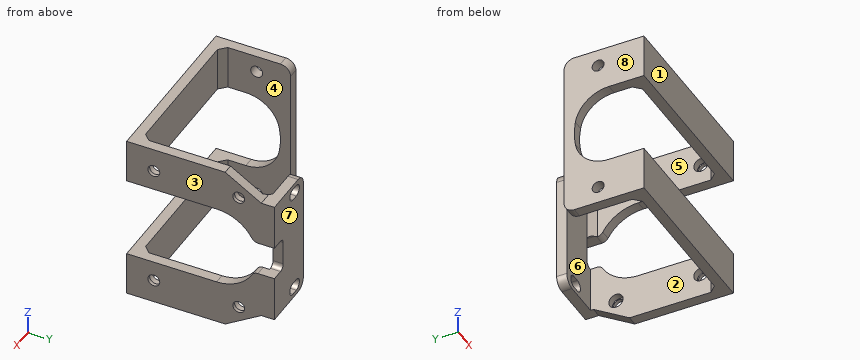
from build123d import *

# Parameters (mm, degrees)
EXTRUDE_THIN1_DEPTH = 25
SKETCH2_R           = 1.75
CUT_EXTRUDE1_DEPTH  = 3
CUT_EXTRUDE2_REACH  = 63.467
CUT_EXTRUDE3_REACH  = 63.467
CUT_EXTRUDE4_DEPTH  = 3
CUT_EXTRUDE5_REACH  = 72.48
SKETCH7_R           = 1.75
FILLET1_R           = 3
CUT_EXTRUDE7_REACH  = 63.467
SKETCH9_R           = 1.75
CUT_EXTRUDE8_START  = -3
CUT_EXTRUDE8_DEPTH  = 3
SKETCH11_R          = 2.1
CUT_EXTRUDE10_DEPTH = 2
CUT_EXTRUDE11_DEPTH = 10
CHAMFER1_SIZE       = 2
FILLET2_R           = 2


with BuildPart() as part:
    # Sketch1 → Extrude-Thin1 (new, symmetric)
    with BuildSketch(Plane.XY):
        Polygon((-1.5, 0), (-1.5, -23.5), (49.5, -23.5), (49.5, 20), (33, 20), (33, 17), (46.5, 17), (46.5, -20.5), (1.5, -20.5), (1.5, 0), align=None)
    extrude(amount=EXTRUDE_THIN1_DEPTH, both=True)

    # Sketch2 → Cut-Extrude1 (cut)
    with BuildSketch(Plane.ZY.offset(1.5)):
        with Locations(Location((-20, -10, 0), (0, 0, 270))):
            Circle(SKETCH2_R)
        with Locations(Location((20, -10, 0), (0, 0, 270))):
            Circle(SKETCH2_R)
    extrude(amount=-CUT_EXTRUDE1_DEPTH, mode=Mode.SUBTRACT)

    # Cut-Extrude2: up to this face of the body (flat: up to its plane)
    cut_extrude2_end = Plane(part.part.faces().sort_by_distance((46.5, -1.75, 0))[0])
    # Sketch3 → Cut-Extrude2 (cut, up to the picked face)
    with BuildSketch(Plane.ZY.offset(1.5), mode=Mode.PRIVATE) as cut_extrude2_sk1:
        with BuildLine():
            Line((-12, -13.167840434), (-12, -27.818696))
            Line((-12, -27.818696), (12, -27.818696))
            Line((12, -27.818696), (12, -13.167840434))
            ThreePointArc((12, -13.167840434), (9.637626158, -6.71286819), (3.666666667, -3.307707462))
            ThreePointArc((3.666666667, -3.307707462), (0, -3), (-3.666666667, -3.307707462))
            ThreePointArc((-3.666666667, -3.307707462), (-9.637626158, -6.71286819), (-12, -13.167840434))
        make_face()
    cut_extrude2_tool1 = split(extrude(cut_extrude2_sk1.sketch, amount=-CUT_EXTRUDE2_REACH, mode=Mode.PRIVATE), bisect_by=cut_extrude2_end, keep=Keep.BOTH, mode=Mode.PRIVATE)
    add(cut_extrude2_tool1.solids().sort_by(Axis((-1.5, -16.267413, 0), (1, 0, 0)))[0], mode=Mode.SUBTRACT)

    # Sketch5 → Cut-Extrude3 (cut, up to next)
    with BuildSketch(Plane(origin=(49.5, 0, 0), x_dir=(0, 0, -1), z_dir=(1, 0, 0)), mode=Mode.PRIVATE) as cut_extrude3_sk1:
        Polygon((-18.5, 20), (-18.5, 16.133851182), (-25, 5.502473915), (-25, 20), align=None)
    cut_extrude3_tool1 = extrude(cut_extrude3_sk1.sketch, amount=-CUT_EXTRUDE3_REACH, mode=Mode.PRIVATE) & part.part
    cut_extrude3 = cut_extrude3_tool1.solids().sort_by_distance((49.5, 14.896175, 22.37718))[0]
    add(cut_extrude3, mode=Mode.SUBTRACT)

    # Mirror1: Cut-Extrude3 across plane
    add(cut_extrude3.mirror(Plane.XY), mode=Mode.SUBTRACT)

    # Sketch6 → Cut-Extrude4 (cut)
    with BuildSketch(Plane(origin=(49.5, 0, 0), x_dir=(0, 0, -1), z_dir=(1, 0, 0))):
        with BuildLine():
            Line((-12, -23.5), (12, -23.5))
            Line((12, -23.5), (12, 3))
            ThreePointArc((12, 3), (0, 15), (-12, 3))
            Line((-12, 3), (-12, -23.5))
        make_face()
    extrude(amount=-CUT_EXTRUDE4_DEPTH, mode=Mode.SUBTRACT)

    # Sketch7 → Cut-Extrude5 (cut, up to next)
    with BuildSketch(Plane(origin=(0, 20, 0), x_dir=(1, 0, 0), z_dir=(0, 1, 0)), mode=Mode.PRIVATE) as cut_extrude5_sk1:
        with Locations(Location((38, 15.5, 0), (0, 0, 180))):
            Circle(SKETCH7_R)
    cut_extrude5_tool1 = extrude(cut_extrude5_sk1.sketch, amount=-CUT_EXTRUDE5_REACH, mode=Mode.PRIVATE) & part.part
    # Sketch7 → Cut-Extrude5 (cut, up to next)
    with BuildSketch(Plane(origin=(0, 20, 0), x_dir=(1, 0, 0), z_dir=(0, 1, 0)), mode=Mode.PRIVATE) as cut_extrude5_sk2:
        with Locations(Location((38, -15.5, 0), (0, 0, 180))):
            Circle(SKETCH7_R)
    cut_extrude5_tool2 = extrude(cut_extrude5_sk2.sketch, amount=-CUT_EXTRUDE5_REACH, mode=Mode.PRIVATE) & part.part
    add(cut_extrude5_tool1.solids().sort_by_distance((38, 20, -15.5))[0], mode=Mode.SUBTRACT)
    add(cut_extrude5_tool2.solids().sort_by_distance((38, 20, 15.5))[0], mode=Mode.SUBTRACT)

    # Fillet1
    fillet1_edges = [part.edges().sort_by_distance(p)[0] for p in [
        (0, 0, 25),
        (33, 18.5, 18.5),
        (0, 0, -25),
        (33, 18.5, -18.5),
    ]]
    fillet(fillet1_edges, radius=FILLET1_R)

    # Sketch9 → Cut-Extrude7 (cut, up to next)
    with BuildSketch(Plane(origin=(49.5, 0, 0), x_dir=(0, 0, -1), z_dir=(1, 0, 0)), mode=Mode.PRIVATE) as cut_extrude7_sk1:
        with Locations((-18, -15.5)):
            Circle(SKETCH9_R)
    cut_extrude7_tool1 = extrude(cut_extrude7_sk1.sketch, amount=-CUT_EXTRUDE7_REACH, mode=Mode.PRIVATE) & part.part
    # Sketch9 → Cut-Extrude7 (cut, up to next)
    with BuildSketch(Plane(origin=(49.5, 0, 0), x_dir=(0, 0, -1), z_dir=(1, 0, 0)), mode=Mode.PRIVATE) as cut_extrude7_sk2:
        with Locations((18, -15.5)):
            Circle(SKETCH9_R)
    cut_extrude7_tool2 = extrude(cut_extrude7_sk2.sketch, amount=-CUT_EXTRUDE7_REACH, mode=Mode.PRIVATE) & part.part
    # Sketch9 → Cut-Extrude7 (cut, up to next)
    with BuildSketch(Plane(origin=(49.5, 0, 0), x_dir=(0, 0, -1), z_dir=(1, 0, 0)), mode=Mode.PRIVATE) as cut_extrude7_sk3:
        with Locations((-18, 9.5)):
            Circle(SKETCH9_R)
    cut_extrude7_tool3 = extrude(cut_extrude7_sk3.sketch, amount=-CUT_EXTRUDE7_REACH, mode=Mode.PRIVATE) & part.part
    # Sketch9 → Cut-Extrude7 (cut, up to next)
    with BuildSketch(Plane(origin=(49.5, 0, 0), x_dir=(0, 0, -1), z_dir=(1, 0, 0)), mode=Mode.PRIVATE) as cut_extrude7_sk4:
        with Locations((18, 9.5)):
            Circle(SKETCH9_R)
    cut_extrude7_tool4 = extrude(cut_extrude7_sk4.sketch, amount=-CUT_EXTRUDE7_REACH, mode=Mode.PRIVATE) & part.part
    add(cut_extrude7_tool1.solids().sort_by_distance((49.5, -15.5, 18))[0], mode=Mode.SUBTRACT)
    add(cut_extrude7_tool2.solids().sort_by_distance((49.5, -15.5, -18))[0], mode=Mode.SUBTRACT)
    add(cut_extrude7_tool3.solids().sort_by_distance((49.5, 9.5, 18))[0], mode=Mode.SUBTRACT)
    add(cut_extrude7_tool4.solids().sort_by_distance((49.5, 9.5, -18))[0], mode=Mode.SUBTRACT)

    # Sketch10 → Cut-Extrude8 (cut)
    with BuildSketch(Plane(origin=(0, 20, 0), x_dir=(1, 0, 0), z_dir=(0, 1, 0)).offset(CUT_EXTRUDE8_START)):
        with BuildLine():
            Line((37, 17.25), (39, 17.25))
            ThreePointArc((39, 17.25), (40.75, 15.5), (39, 13.75))
            Line((39, 13.75), (37, 13.75))
            ThreePointArc((37, 13.75), (35.25, 15.5), (37, 17.25))
        make_face()
        with BuildLine():
            Line((37, -13.75), (39, -13.75))
            ThreePointArc((39, -13.75), (40.75, -15.5), (39, -17.25))
            Line((39, -17.25), (37, -17.25))
            ThreePointArc((37, -17.25), (35.25, -15.5), (37, -13.75))
        make_face()
    extrude(amount=CUT_EXTRUDE8_DEPTH, mode=Mode.SUBTRACT)

    # Sketch11 → Cut-Extrude10 (cut)
    with BuildSketch(Plane.ZY.offset(-46.5)):
        with Locations((-18, 9.5)):
            Circle(SKETCH11_R)
        with Locations((18, 9.5)):
            Circle(SKETCH11_R)
        with Locations((18, -15.5)):
            Circle(SKETCH11_R)
        with Locations((-18, -15.5)):
            Circle(SKETCH11_R)
    extrude(amount=-CUT_EXTRUDE10_DEPTH, mode=Mode.SUBTRACT)

    # Sketch12 → Cut-Extrude11 (cut)
    with BuildSketch(Plane(origin=(0, 20, 0), x_dir=(1, 0, 0), z_dir=(0, 1, 0))):
        with BuildLine():
            Line((49.5, -5), (46, -5))
            ThreePointArc((46, -5), (44.939339828, -4.560660172), (44.5, -3.5))
            Line((44.5, -3.5), (44.5, 3.5))
            ThreePointArc((44.5, 3.5), (44.939339828, 4.560660172), (46, 5))
            Line((46, 5), (49.5, 5))
            Line((49.5, 5), (49.5, -5))
        make_face()
    extrude(amount=-CUT_EXTRUDE11_DEPTH, mode=Mode.SUBTRACT)

    # Chamfer1
    chamfer1_edges = [part.edges().sort_by_distance(p)[0] for p in [
        (46.5, 17, 11.75),
        (1.5, -20.5, -18.5),
        (1.5, -20.5, 18.5),
        (46.5, -20.5, 18.5),
        (46.5, -20.5, -18.5),
    ]]
    chamfer(chamfer1_edges, length=CHAMFER1_SIZE - 0.0001)  # a hair under: the kernel refuses the full size

    # Fillet2
    fillet2_edges = [part.edges().sort_by_distance(p)[0] for p in [
        (48, 13.908712115, -5),
        (48, 13.908712115, 5),
    ]]
    fillet(fillet2_edges, radius=FILLET2_R)


solid = part.part
Work out the finished part from the listing and answer in its coordinate system (mm). Face numbers are marked on the shaded views. A direction names the side the tool comes from. Give positions to 0.01 mm unless a question says otherwise; leave off trailing zeros. Loops run counter-clockwise (first coordinate to the right, second up) from the corner with the lowest first, then second, coordinate; pieces in that order, holes last. Notation, with made-up numbers: (64.5, -27) -> (90.5, -27) arc R12 cw to (90.5, -19) -> close; hole circle Ø4 at (80, -36.75). An arc over 180 degrees is marked (long way). Use a Markdown table: item, result. Add a question column.
1. Section D-D on z = 8 is taken. Determine the outline of the cut face in (x, y), and give its area (3 significant figures).
2. Flat-ended cylindrical pins translate along their axes: pin 1 Ø2 at (x, y) = (38, 18.5) entering from +Z; pin 2 Ø12 at (x, y) = (29.5, -10.5) entering from -Z; pin 3 Ø3 at (x, y) = (47.5, 16.5) entering from -Z; pin 4 Ø6.5 at (x, z) = (26.5, 19.5) entering from +Y. Find the tip coordinate at first contact, or state that the pin passes through.
3. For the marked faces 1, 2, 3, 4 and 5, determine the directions among +Z, -Z, +X, -X, +Y, -Y from which every point of the face is accessible in a straight line to the end or side of a thin tool.
4. Find the intervals of material crossed by probe 1 along Y at (x, z) = (47.5, 18); probe 2 along X at (y, z) = (-17, 22); probe 3 along Z at (x, y) = (47, 9), in increasing order.
5. Section C-C on x = 42 is taken. Determine the outline of the cut face in (y, z), and give its area (3 significant figures).
6. Section B-B on y = 1 is taken. Determine the outline of the cut face in (x, z), and give its area (3 significant figures).
7. Determine the mould class of the marked faces 6, 7 and 8 for opening direction Y: released by +Y, released by -Y, zero draft, split by the parting line, or undercut.
8. Section A-A on x = 7 is taken. Determine the outline of the cut face in (y, z), and give its area (3 significant figures).
Results below:
| question | item | result |
|---|---|---|
| 1 | outline | (-1.5, -5.17) -> (1.5, -5.17) -> (1.5, 0) -> (-1.5, 0) -> close; (33, 17) -> (44.5, 17) -> (46.5, 15) -> (46.5, 11.94) -> (49.5, 11.94) -> (49.5, 20) -> (33, 20) -> close |
| 1 | area | 82.2 mm^2 |
| 2 | pin 1 | stops at z = 18.5 |
| 2 | pin 2 | passes through |
| 2 | pin 3 | stops at z = -19.19 |
| 2 | pin 4 | stops at y = -20.5 |
| 3 | face 1 | +Z, -Z, +X, -X, -Y |
| 3 | face 2 | -Z |
| 3 | face 3 | +Z, -Z, +X, +Y, -Y |
| 3 | face 4 | +Z, -Z, +Y |
| 3 | face 5 | +Z, -Z |
| 4 | probe 1 | y = -23.5 to -17.6, -13.4 to 7.4, 11.6 to 20 |
| 4 | probe 2 | x = -1.5 to 1.5, 46.5 to 49.5 |
| 4 | probe 3 | z = -22.86 to -20.04, -15.96 to -10.39, 10.39 to 15.96, 20.04 to 22.86 |
| 5 | outline | (-23.5, -25) -> (-20.5, -25) -> (-20.5, -12) -> (-23.5, -12) -> close; (-23.5, 12) -> (-20.5, 12) -> (-20.5, 25) -> (-23.5, 25) -> close; (17, -18.5) -> (20, -18.5) -> (20, 18.5) -> (17, 18.5) -> close |
| 5 | area | 189 mm^2 |
| 6 | outline | (46.5, -25) -> (49.5, -25) -> (49.5, -12) -> (46.5, -12) -> close; (46.5, 12) -> (49.5, 12) -> (49.5, 25) -> (46.5, 25) -> close |
| 6 | area | 78.0 mm^2 |
| 7 | face 6 | undercut |
| 7 | face 7 | released by +Y |
| 7 | face 8 | zero draft |
| 8 | outline | (-23.5, -25) -> (-20.5, -25) -> (-20.5, -12) -> (-23.5, -12) -> close; (-23.5, 12) -> (-20.5, 12) -> (-20.5, 25) -> (-23.5, 25) -> close |
| 8 | area | 78.0 mm^2 |
